Source: CAD feature listing. Evaluate the final solid. Frame: model axes, mm. A direction names the side the tool comes from. Give positions to 0.01 mm unless a question says otherwise; leave off trailing zeros. Loops run counter-clockwise (first coordinate to the right, second up) from the corner with the lowest first, then second, coordinate; pieces in that order, holes last. Notation, with made-up numbers: (-25.5, 38) -> (-17.5, 38) arc R21 ccw to (-17.5, 73) -> close; hole circle Ø1 at (65.25, 84). An arc over 180 degrees is marked (long way). Put each result on its own line as item: value.
Autodesk Fusion 360 part; units mm, degrees
box "BoxPrimitive1" add length 280 width 560 height 250 placed x (0, 1, 0) y (-1, 0, 0) z (0, 0, 1) at (560, 0, 0)
sketch "Sketch2" plane through (560, 0, 0) normal (1, 0, 0) x (0, 1, 0)
  line L0 (0, 250) -> (0, 0)
  line L1 (0, 0) -> (280, 0)
  line L2 (280, 0) -> (280, 250)
  line L3 (280, 250) -> (0, 250)
  line L4 (0, 0) -> (230, 250)
  line L5 (193.2, 210) -> (280, 210)
  line L6 (147.2, 160) -> (0, 160)
  dimension "d6" = 50
  dimension "d7" = 160
  dimension "d8" = 50
extrude "Extrude1" cut sketch "Sketch2" against normal blind 560 contours L0 L3 L4 L6
extrude "Extrude2" cut sketch "Sketch2" against normal blind 400 from surface at -80 contours L0 L4 L6
extrude "Extrude3" cut sketch "Sketch2" against normal blind 120 contours L2 L3 L4 L5
ref_plane "WorkPlane1" through (280, 140, 105) normal (1, 0, 0) x (0, 0, -1)
mirror "Mirror1" about plane through (280, 140, 105) normal (1, 0, 0) of "Extrude3"
sketch "Sketch3" plane through (0, 0, 0) normal (0, -0.7359, 0.6771) x (1, 0, 0)
  line L0 (120, 285.3528) -> (0, 285.3528)
  line L1 (0, 285.3528) -> (0, 217.4117)
  line L2 (0, 217.4117) -> (80, 217.4117)
  line L3 (80, 217.4117) -> (80, 0)
  line L4 (80, 0) -> (480, 0)
  line L5 (480, 0) -> (480, 217.4117)
  line L6 (480, 217.4117) -> (560, 217.4117)
  line L7 (560, 217.4117) -> (560, 285.3528)
  line L8 (560, 285.3528) -> (440, 285.3528)
  line L9 (440, 285.3528) -> (440, 339.7058)
  line L10 (440, 339.7058) -> (120, 339.7058)
  line L11 (120, 339.7058) -> (120, 285.3528)
  line L12 (360, 80) -> (200, 80)
  line L13 (200, 80) -> (200, 240)
  line L14 (200, 240) -> (360, 240)
  line L15 (360, 240) -> (360, 80)
  line L16 (360, 80) -> (200, 240) construction
  line L17 (200, 80) -> (360, 240) construction
  point P0 (280, 160)
  dimension "d18" = 160
  dimension "d19" = 160
  dimension "d20" = 80
  dimension "d21" = 120
sketch "Sketch4" plane through (0, 280, 0) normal (0, 1, 0) x (-1, 0, 0)
  line L0 (0, 210) -> (-120, 210)
  line L1 (-120, 210) -> (-120, 250)
  line L2 (-120, 250) -> (-440, 250)
  line L3 (-440, 250) -> (-440, 210)
  line L4 (-440, 210) -> (-560, 210)
  line L5 (-560, 210) -> (-560, 0)
  line L6 (-560, 0) -> (0, 0)
  line L7 (0, 0) -> (0, 210)
  line L8 (-200, 58.8745) -> (-200, 176.6234)
  line L9 (-200, 176.6234) -> (-360, 176.6234)
  line L10 (-360, 58.8745) -> (-200, 58.8745)
  line L11 (-360, 176.6234) -> (-360, 58.8745)
extrude "Extrude4" cut sketch "Sketch4" against normal blind 300 contours L8 L9 L10 L11
(1) Section D-D on y = 204. Return loops of the section in (x, z).
Calculated:
outline: (0, 0) -> (560, 0) -> (560, 210) -> (440, 210) -> (440, 221.74) -> (120, 221.74) -> (120, 210) -> (0, 210) -> close; hole (200, 58.87) -> (360, 58.87) -> (360, 176.62) -> (200, 176.62) -> close
(2) Section C-C on z = 45. Return loops of the section in (x, y), then the cut area to 3 significant figures.
Calculated:
outline: (0, 0) -> (80, 0) -> (80, 41.4) -> (480, 41.4) -> (480, 0) -> (560, 0) -> (560, 280) -> (0, 280) -> close
area: 140,000 mm²
(3) First-contact query: P1, Ø3, axis at x = 96, z = 111.5, coming from the -Y side; P2, Ø24, axis at x = 518.5, y = 59.5, coming from the +Z side. Flat tips, straight axial feed; report the tip coordinate or a pass-through.
Calculated:
P1: stops at y = 101.2
P2: stops at z = 160
(4) Section B-B on x = 225. Return loops of the section in (y, z).
Calculated:
outline: (0, 0) -> (280, 0) -> (280, 58.87) -> (54.16, 58.87) -> close; (162.49, 176.62) -> (280, 176.62) -> (280, 250) -> (230, 250) -> close
(5) Section A-A on z = 123. Return loops of the section in (x, y), then the cut area to 3 significant figures.
Calculated:
outline: (0, 0) -> (80, 0) -> (80, 113.16) -> (200, 113.16) -> (200, 280) -> (0, 280) -> close; (360, 113.16) -> (480, 113.16) -> (480, 0) -> (560, 0) -> (560, 280) -> (360, 280) -> close
area: 84,800 mm²
(6) Draft query along X for faces 6 (the flat face through (200, 194, 117)), 7 (the flat face through (59, 237, 210)), 8 (the flat face through (80, 56, 99)), 9 (the flat face through (0, 142, 80)). Return one class per face: released by +X, released by -X, zero draft, split by the parting line, or undercut.
Calculated:
face 6: undercut
face 7: zero draft
face 8: undercut
face 9: released by -X
(7) Line query: probe 1 along Z at (x, y) = (283, 241.5); probe 2 along X at (y, z) = (77, 151.5); probe 3 along Z at (x, y) = (75.5, 40). Output: solid intervals per line, ascending. Write a range as from..to.
Calculated:
probe 1: z = 0..58.87, 176.62..250
probe 2: x = 0..80, 480..560
probe 3: z = 0..160
(8) Reachability of faces 1 (the flat face through (278, 255, 250)), 2 (the flat face through (521, 75, 160)), 3 (the flat face through (480, 56, 99)), 4 (the flat face through (281, 169, 58.874)), 5 (the flat face through (440, 246, 230)) from +Z, -Z, +X, -X, +Y, -Y: full face, straight path, thin tool, end or side. Return the list, or none.
Calculated:
face 1: +Z, +X, -X, +Y, -Y
face 2: +Z, +X, -X, -Y
face 3: +Z, -Y
face 4: +Y, -Y
face 5: +Z, +X, +Y, -Y
